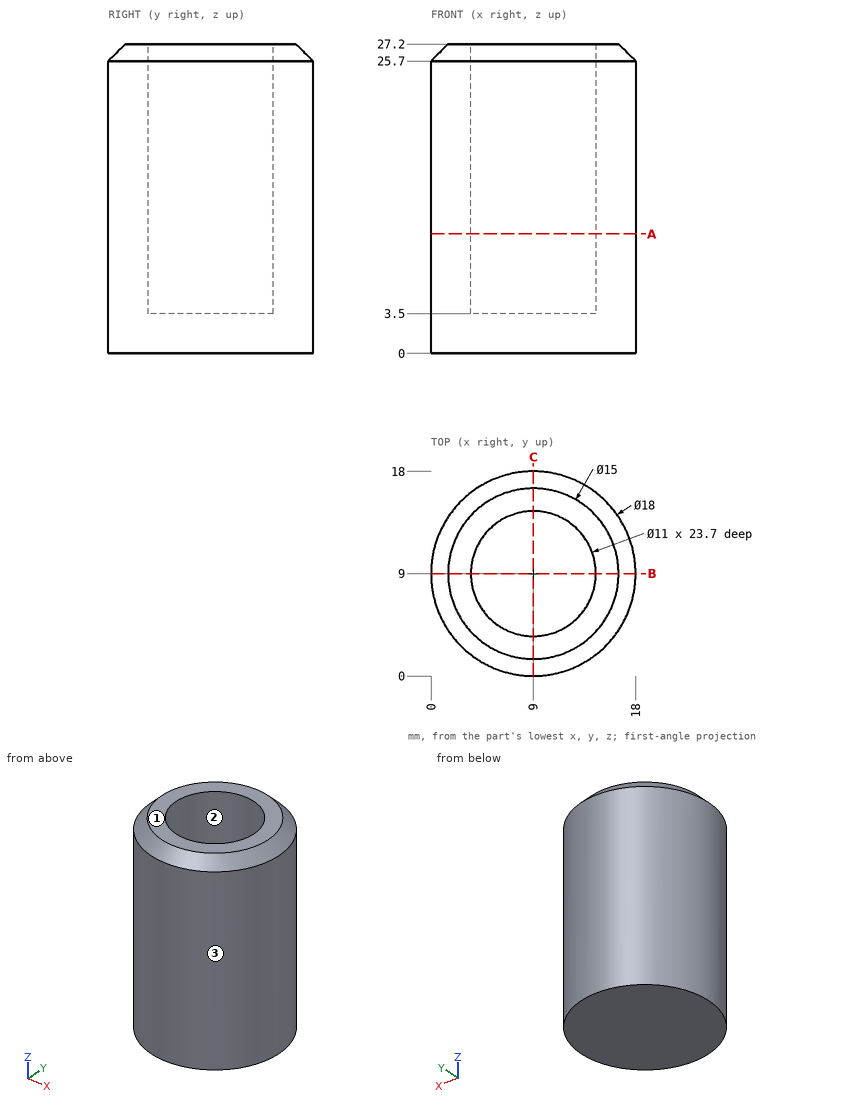
Could you check a few things on this drawing? It's one solid part, dimensions in mm from its lowest x, y, z. Coordinates: 2 decimals unless noted, no trailing zeros. Write each loop counter-clockwise with the first axis right and the second up, starting at its lowest first coordinate (ties: lowest second). Pieces come first, ordered by that corner, then holes. Notation, with made-up numbers: (-8.75, 22.5) - (3.25, 22.5) arc R25 cw to (3.25, 58.5) - close; hole circle Ø10 at (-2.5, 27.5). An arc over 180 degrees is marked (long way). Write item = value, one per line.
1) Suppose I cut it at B-B on y = 9. Please give me the cut outline in (x, z), plus the area to 3 significant figures.
Result set:
outline = (0, 0) - (18, 0) - (18, 25.7) - (16.5, 27.2) - (14.5, 27.2) - (14.5, 3.5) - (3.5, 3.5) - (3.5, 27.2) - (1.5, 27.2) - (0, 25.7) - close
area = 227 mm2
2) Please list where these lines run through material, in increasing order: line 1 (Y direction, x = 9, z = 12.75); line 2 (Z direction, x = 9.5, y = 8); line 3 (X direction, y = 6.5, z = 4.5). Write a range as [from, to].
Result set:
line_1 = [0, 3.5], [14.5, 18]
line_2 = [0, 3.5]
line_3 = [0.35, 4.1], [13.9, 17.65]
3) Will these pins go through, and if not, where does the flat tip stop? pin 1 Ø2 at (x, y) = (10, 16) entering from -Z; pin 2 Ø4 at (y, z) = (3.5, 22) entering from -X; pin 3 Ø5 at (x, z) = (6, 21.5) entering from +Y; pin 4 Ø8 at (y, z) = (15.5, 6.5) entering from +X.
Result set:
pin_1 = 0
pin_2 = 0.71
pin_3 = 17.99
pin_4 = 17.65
4) Suppose I cut it at A-A on z = 10.5. Please give me the cut outline in (x, y), plus the area to 3 significant figures.
Result set:
outline = circle Ø18 at (9, 9); hole circle Ø11 at (9, 9)
area = 159 mm2
5) We'd pull the mould along Y, two halves only. Please class the marked faces 1, 2 and 3: +Y half, -Y half, draft (parallel to the pull), parting line (faces both ways), or undercut.
Result set:
face_1 = draft
face_2 = undercut
face_3 = parting line
